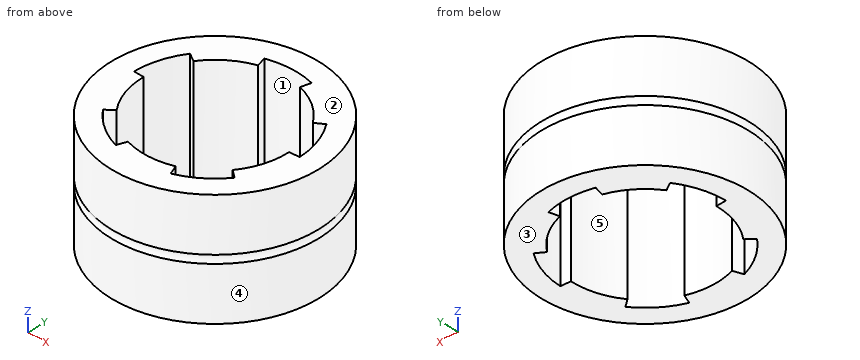
from build123d import *

# Parameters (mm, degrees)
SKETCH1_R           = 30.75
BOSS_EXTRUDE1_DEPTH = 34


with BuildPart() as part:
    # Sketch1 → Boss-Extrude1 (new body)
    with BuildSketch(Plane.XY):
        Circle(SKETCH1_R)
        with BuildLine():
            Line((-17.649126209, 12.27836895), (-20.165137913, 13.912286055))
            ThreePointArc((-20.165137913, 13.912286055), (-23.299613116, 7.570503216), (-24.491375834, 0.597494827))
            Line((-24.491375834, 0.597494827), (-21.49548723, 0.440486958))
            ThreePointArc((-21.49548723, 0.440486958), (-20.4477151, -6.643865379), (-17.131302733, -12.991091819))
            Line((-17.131302733, -12.991091819), (-19.462740618, -14.879052992))
            ThreePointArc((-19.462740618, -14.879052992), (-14.39995283, -19.819834732), (-8.136502697, -23.108046524))
            Line((-8.136502697, -23.108046524), (-7.061398848, -20.307305245))
            ThreePointArc((-7.061398848, -20.307305245), (0, -21.5), (7.061398848, -20.307305245))
            Line((7.061398848, -20.307305245), (8.136502697, -23.108046524))
            ThreePointArc((8.136502697, -23.108046524), (14.39995283, -19.819834732), (19.462740618, -14.879052992))
            Line((19.462740618, -14.879052992), (17.131302733, -12.991091819))
            ThreePointArc((17.131302733, -12.991091819), (20.4477151, -6.643865379), (21.49548723, 0.440486958))
            Line((21.49548723, 0.440486958), (24.491375834, 0.597494827))
            ThreePointArc((24.491375834, 0.597494827), (23.299613116, 7.570503216), (20.165137913, 13.912286055))
            Line((20.165137913, 13.912286055), (17.649126209, 12.27836895))
            ThreePointArc((17.649126209, 12.27836895), (12.637382924, 17.393865379), (6.223542865, 20.579541156))
            Line((6.223542865, 20.579541156), (7, 23.477318635))
            ThreePointArc((7, 23.477318635), (0, 24.498663031), (-7, 23.477318635))
            Line((-7, 23.477318635), (-6.223542865, 20.579541156))
            ThreePointArc((-6.223542865, 20.579541156), (-12.637382924, 17.393865379), (-17.649126209, 12.27836895))
        make_face(mode=Mode.SUBTRACT)
    extrude(amount=-BOSS_EXTRUDE1_DEPTH)

    # Sketch2 → Cut-Revolve1 (revolve, cut)
    with BuildSketch(Plane.ZY):
        with BuildLine():
            Line((-18.2, 30.75), (-15.8, 30.75))
            ThreePointArc((-15.8, 30.75), (-17, 30.25), (-18.2, 30.75))
        make_face()
    revolve(axis=Axis((0, 0, 27.953503857), (0, 0, -1)), mode=Mode.SUBTRACT)


solid = part.part
Design review of the part built by this model. Coordinates are the model's own, in mm. Face numbers are marked on the shaded views. A direction names the side the tool comes from. Round coordinates to 2 decimals unless told otherwise and drop trailing zeros. Order: outer loops, then holes, each group sorted by start corner. A loop starts at its lowest first (then second) coordinate and runs counter-clockwise, first axis right, second up.
1) Consider section C-C (x = -18.5). Count the separate pieces of the cut face and the enclosed holes in it, plus the area to 3 significant figures.
The answers:
separate pieces: 3
enclosed holes: 0
area: 793 mm2
2) Draft analysis for pull direction X (two halves, no side actions). For the marked faces 3, 4 and 5, state which applies: released by +X, released by -X, zero draft, split by the parting line, or undercut.
The answers:
face 3: zero draft
face 4: split by the parting line
face 5: undercut
3) Machinability: for the marked faces 1 and 2, which of the approach directions +Z, -Z, +X, -X, +Y, -Y give a long, thin tool a straight path to every point of the face, cutting with its end or side? Answer none if there is none.
The answers:
face 1: +Z, -Z
face 2: +Z, +X, -X, +Y, -Y
4) For L1, parallel to Y at x = -1, z = -7; L2, parallel to Y at x = 18, z = -30.5; L3, parallel to Y at x = 14, z = -16.5, list the stretches that pass through material, from the lowest coordinate up.
The answers:
L1: y = -30.73 to -21.48, 24.48 to 30.73
L2: y = -24.93 to -16.62, -13.69 to -11.76, 12.51 to 24.93
L3: y = -26.9 to -20.1, 16.32 to 26.9
5) Consider section B-B (z = -21.5). State the section outline as (x, y) points, plus the area to 3 significant figures.
The answers:
outline: circle Ø61.5 at (0, 0); hole (-24.49, 0.6) - (-21.5, 0.44) arc R21.5 ccw to (-17.13, -12.99) - (-19.46, -14.88) arc R24.5 ccw to (-8.14, -23.11) - (-7.06, -20.31) arc R21.5 ccw to (7.06, -20.31) - (8.14, -23.11) arc R24.5 ccw to (19.46, -14.88) - (17.13, -12.99) arc R21.5 ccw to (21.5, 0.44) - (24.49, 0.6) arc R24.5 ccw to (20.17, 13.91) - (17.65, 12.28) arc R21.5 ccw to (6.22, 20.58) - (7, 23.48) arc R24.5 ccw to (-7, 23.48) - (-6.22, 20.58) arc R21.5 ccw to (-17.65, 12.28) - (-20.17, 13.91) arc R24.5 ccw to start
area: 1,320 mm2
6) Clearance check with flat-ended pins moving along their axes: pin 1 Ø8 at (y, z) = (2, -5.5) entering from +X; pin 2 Ø8 at (x, y) = (16, 2) entering from -Z (3 decimals); pin 3 Ø6 at (y, z) = (10.5, -19) entering from +X; pin 4 Ø6 at (x, z) = (-5, -11) entering from -Y. State where each tip first meets the part, or that it passes through.
The answers:
pin 1: stops at x = 30.75
pin 2: passes through
pin 3: stops at x = 29.82
pin 4: stops at y = -30.68
7) Consider section A-A (x = 0). State the section outline as (y, z) points.
The answers:
outline: (-30.75, -34) - (-21.5, -34) - (-21.5, 0) - (-30.75, 0) - (-30.75, -15.8) arc R1.69 cw to (-30.75, -18.2) - close; (24.5, -34) - (30.75, -34) - (30.75, -18.2) arc R1.69 cw to (30.75, -15.8) - (30.75, 0) - (24.5, 0) - close
